Geometry check sheet. Reference: the model listing, model coordinates, mm. Face numbers are marked on the shaded views. A direction names the side the tool comes from. Give positions to 0.01 mm unless a question says otherwise; leave off trailing zeros. Order: outer loops, then holes, each group sorted by start corner. A loop starts at its lowest first (then second) coordinate and runs counter-clockwise, first axis right, second up. Notation, with made-up numbers: M -19,17.25 L 35,17.25 A18 cw 35,50.25 Z; hole C 8,-14 d4. An arc over 180 degrees is marked long. Answer as CSV lines item,"result". Start each with the question number.
Q1. Thickness scan on line 1 (Y direction, x = 5, z = 2.9); line 2 (Y direction, x = 35, z = 1.65); line 3 (Y direction, x = 20, z = 2.4). Record the ranges inside material, lowest first.
Q2. Section check B-B, the plane z = 3.25. Record the boundary of the cut face in (x, y).
Q3. Set-up check for the marked faces 4, 5, 6 and 7: record each of +Z, -Z, +X, -X, +Y, -Y from which the full face is reachable in a straight line by a thin tool's end or side.
Q4. Mould release check, pull along X, two halves, no side actions. Record for the marked faces 1, 2 and 3: +X half, -X half, draft (parallel to the pull), parting line (faces both ways), or undercut.
Q5. Go/stop test with flat-tipped pins: pin 1 (1 mm diameter, centred on x = 14.5, z = 7, fed in from +Y); pin 2 (4 mm diameter, centred on x = 26, z = 6.5, fed in from -Y); pin 3 (7 mm diameter, centred on x = 5, y = 5, fed in from +Z); pin 4 (1.8 mm diameter, centred on x = 5, y = 5, fed in from +Z). Record where each tip stops, or that it passes through.
Q6. Section check D-D, the plane x = 20. Record the boundary of the cut face in (y, z).
Q7. Section check C-C, the plane y = 15. Record the boundary of the cut face in (x, z), then the cut area to 3 significant figures.
Q8. Section check A-A, the plane x = 35. Record the boundary of the cut face in (y, z).
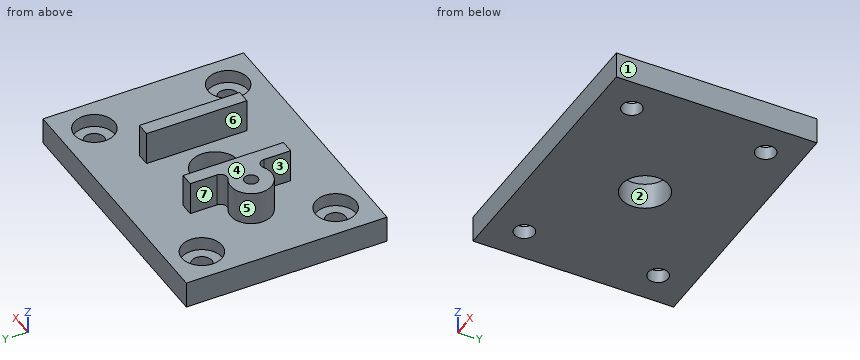
```python
from build123d import *

# Parameters (mm, degrees)
SKIZZE1_W                       = 40
SKIZZE1_H                       = 30
SKIZZE1_R                       = 3.5
SKIZZE1_R_2                     = 3
AUFSATZ_LINEAR_AUSTRAGEN1_DEPTH = 4
SKIZZE1_3_R                     = 3
SKIZZE1_3_R_2                   = 1.5
AUFSATZ_LINEAR_AUSTRAGEN2_DEPTH = 2
SKIZZE2_R                       = 3.05
SKIZZE2_R_2                     = 1
AUFSATZ_LINEAR_AUSTRAGEN5_DEPTH = 5
VERRUNDUNG1_R                   = 1


with BuildPart() as part:
    # Skizze1 → Aufsatz-Linear austragen1 (new body)
    with BuildSketch(Plane.XY):
        with Locations((20, 15)):
            Rectangle(SKIZZE1_W, SKIZZE1_H)
        with Locations((20, 15)):
            Circle(SKIZZE1_R, mode=Mode.SUBTRACT)
        with Locations((5, 25)):
            Circle(SKIZZE1_R_2, mode=Mode.SUBTRACT)
        with Locations((35, 25)):
            Circle(SKIZZE1_R_2, mode=Mode.SUBTRACT)
        with Locations((35, 5)):
            Circle(SKIZZE1_R_2, mode=Mode.SUBTRACT)
        with Locations((5, 5)):
            Circle(SKIZZE1_R_2, mode=Mode.SUBTRACT)
    extrude(amount=AUFSATZ_LINEAR_AUSTRAGEN1_DEPTH)

    # Skizze1_3 → Aufsatz-Linear austragen2 (add)
    with BuildSketch(Plane.XY):
        with Locations((5, 25)):
            Circle(SKIZZE1_3_R)
        with Locations((5, 25)):
            Circle(SKIZZE1_3_R_2, mode=Mode.SUBTRACT)
        with Locations((35, 25)):
            Circle(SKIZZE1_3_R)
        with Locations((35, 25)):
            Circle(SKIZZE1_3_R_2, mode=Mode.SUBTRACT)
        with Locations((35, 5)):
            Circle(SKIZZE1_3_R)
        with Locations((35, 5)):
            Circle(SKIZZE1_3_R_2, mode=Mode.SUBTRACT)
        with Locations((5, 5)):
            Circle(SKIZZE1_3_R)
        with Locations((5, 5)):
            Circle(SKIZZE1_3_R_2, mode=Mode.SUBTRACT)
    extrude(amount=AUFSATZ_LINEAR_AUSTRAGEN2_DEPTH)

    # Skizze2 → Aufsatz-Linear austragen5 (add)
    with BuildSketch(Plane.XY.offset(4)):
        with Locations((9.9, 15)):
            Circle(SKIZZE2_R)
        with Locations((9.9, 15)):
            Circle(SKIZZE2_R_2, mode=Mode.SUBTRACT)
        Polygon((14.9, 15), (14.9, 22.5), (12.9, 22.5), (12.9, 7.5), (14.9, 7.5), align=None)
        Polygon((25.1, 7.5), (25.1, 15), (25.1, 22.5), (27.1, 22.5), (27.1, 7.5), align=None)
    extrude(amount=AUFSATZ_LINEAR_AUSTRAGEN5_DEPTH)

    # Verrundung1
    verrundung1_edges = [part.edges().sort_by_distance(p)[0] for p in [
        (12.9, 15.55, 6.5),
        (12.9, 14.45, 6.5),
    ]]
    fillet(verrundung1_edges, radius=VERRUNDUNG1_R)


solid = part.part
```
Answer block:
1,line 1,"y = 0 to 2, 8 to 22, 28 to 30"
1,line 2,"y = 0 to 3.5, 6.5 to 23.5, 26.5 to 30"
1,line 3,"y = 0 to 11.5, 18.5 to 30"
2,outline,"M 0,0 L 40,0 L 40,30 L 0,30 Z; hole C 5,5 d6; hole C 5,25 d6; hole C 20,15 d7; hole C 35,5 d6; hole C 35,25 d6"
3,face 4,"+Z, +X, -X, +Y, -Y"
3,face 5,"+Z"
3,face 6,"+Z, +Y, -Y"
3,face 7,"+Z, -X, +Y"
4,face 1,"+X half"
4,face 2,"undercut"
4,face 3,"-X half"
5,pin 1,"stops at y = 22.5"
5,pin 2,"stops at y = 7.5"
5,pin 3,"stops at z = 4"
5,pin 4,"passes through"
6,outline,"M 0,0 L 11.5,0 L 11.5,4 L 0,4 Z; M 18.5,0 L 30,0 L 30,4 L 18.5,4 Z"
7,outline,"M 0,0 L 16.5,0 L 16.5,4 L 14.9,4 L 14.9,9 L 10.9,9 L 10.9,4 L 8.9,4 L 8.9,9 L 6.85,9 L 6.85,4 L 0,4 Z; M 23.5,0 L 40,0 L 40,4 L 27.1,4 L 27.1,9 L 25.1,9 L 25.1,4 L 23.5,4 Z"
7,area,"172 mm2"
8,outline,"M 0,0 L 3.5,0 L 3.5,2 L 2,2 L 2,4 L 0,4 Z; M 6.5,0 L 23.5,0 L 23.5,2 L 22,2 L 22,4 L 8,4 L 8,2 L 6.5,2 Z; M 26.5,0 L 30,0 L 30,4 L 28,4 L 28,2 L 26.5,2 Z"
